Design review of the part built by this model. Coordinates are the model's own, in mm. Face numbers are marked on the shaded views. A direction names the side the tool comes from. Round coordinates to 2 decimals unless told otherwise and drop trailing zeros. Write each loop counter-clockwise with the first axis right and the second up, starting at its lowest first coordinate (ties: lowest second). Pieces come first, ordered by that corner, then holes.
from build123d import *

# Parameters (mm, degrees)
SKETCH1_W               = 6426.2
SKETCH1_H               = 2311.4
BOSS_EXTRUDE1_DEPTH     = 3175
SKETCH2_R               = 763.27
CUT_EXTRUDE1_DEPTH      = 2057.4
CUT_EXTRUDE3_DEPTH      = 7475.536972742
CUT_EXTRUDE3_DEPTH_BACK = 7475.536972742
SKETCH6_W               = 1295.4
SKETCH6_H               = 1651
CUT_EXTRUDE4_DEPTH      = 7523.97968682
CUT_EXTRUDE4_DEPTH_BACK = 7523.97968682
SKETCH7_R               = 444.5
SCALE1_SCALE            = 0.039370079


with BuildPart() as part:
    # Sketch1 → Boss-Extrude1 (new body)
    with BuildSketch(Plane(origin=(0, 0, 0), x_dir=(1, 0, 0), z_dir=(0, 1, 0))):
        with Locations((3156.321169036, 1128.715007899)):
            Rectangle(SKETCH1_W, SKETCH1_H)
    extrude(amount=BOSS_EXTRUDE1_DEPTH)

    # Sketch2 → Cut-Extrude1 (cut)
    with BuildSketch(Plane(origin=(0, 3175, 0), x_dir=(1, 0, 0), z_dir=(0, 1, 0))):
        with Locations(Location((1098.921169036, 1128.715007899, 0), (0, 0, 270))):
            Circle(SKETCH2_R)
        with Locations(Location((3156.321169036, 1128.715007899, 0), (0, 0, 270))):
            Circle(SKETCH2_R)
        with Locations(Location((5213.721169036, 1128.715007899, 0), (0, 0, 270))):
            Circle(SKETCH2_R)
    extrude(amount=-CUT_EXTRUDE1_DEPTH, mode=Mode.SUBTRACT)

    # Sketch6 → Cut-Extrude3 (cut, two sides: drawn at the far end of the back side and taken through both)
    with BuildSketch(Plane.XY.offset(-CUT_EXTRUDE3_DEPTH_BACK)):
        with Locations((3156.321169036, 818.341718397)):
            Rectangle(SKETCH6_W, SKETCH6_H)
        with Locations((5213.721169036, 825.5)):
            Rectangle(SKETCH6_W, SKETCH6_H)
        with Locations((1098.921169036, 825.5)):
            Rectangle(SKETCH6_W, SKETCH6_H)
    extrude(amount=CUT_EXTRUDE3_DEPTH + CUT_EXTRUDE3_DEPTH_BACK, mode=Mode.SUBTRACT)

    # Sketch7 → Cut-Extrude4 (cut, two sides: drawn at the far end of the back side and taken through both)
    with BuildSketch(Plane(origin=(6369.421169036, 0, 0), x_dir=(0, 0, -1), z_dir=(1, 0, 0)).offset(-CUT_EXTRUDE4_DEPTH_BACK)):
        with Locations((1128.715007899, 0)):
            Circle(SKETCH7_R)
    extrude(amount=CUT_EXTRUDE4_DEPTH + CUT_EXTRUDE4_DEPTH_BACK, mode=Mode.SUBTRACT)


with BuildPart() as part_1:
    # Scale1: scaled about (0, 0, 0)
    add(part.part.scale(SCALE1_SCALE))


solid = part_1.part
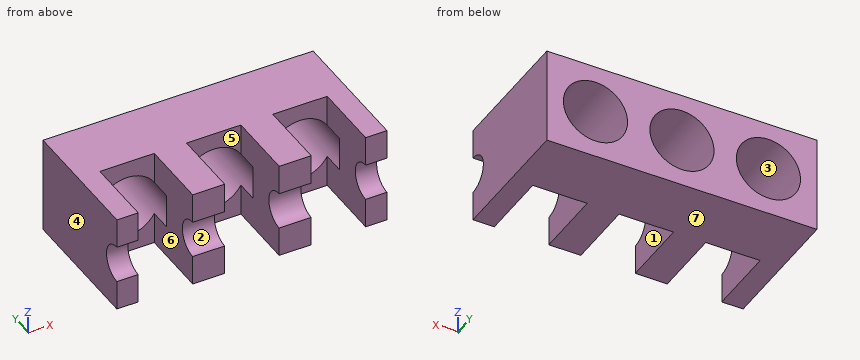
1) Add section B-B on x = 24. State the section outline as (y, z) points.
2) Add section C-C on z = -49. State the section outline as (x, y) points, and give its area (3 significant figures).
3) For the marked faces 1, 2 and 3, list the 3-axis set-ups (+Z, -Z, +X, -X, +Y, -Y) from which the entire face can be reached by the end or side of a thin tool; tool diameter is ignored.
4) For line 1 along X through (y, z) = (60, -22); line 2 along X through (y, z) = (116.5, -63.5); line 3 along Z through (x, y) = (178.5, 9), list the stretches that pass through material, from the lowest coordinate up.
5) Add section A-A on y = 60. State the section outline as (x, z) points.
6) For P1, Ø9, axis at x = 52.5, z = -9, coming from the -Y side; P2, Ø2.5, axis at x = 16, z = -39, coming from the +Y side; P3, Ø5, axis at x = 97.5, z = -51.5, coming from the +Y side; P4, Ø9, axis at x = 119.5, z = -11.5, coming from the -Y side, all flat-tipped, find the tip position at first contact; note any pin that passes through.
7) Add section D-D on x = 91. State the section outline as (y, z) points, and give its area (3 significant figures).
8) The part is to be moulded in two halves that separate along X. For the marked faces 4, 5, 6 and 7, say which applies: pulls with the +X half, pulls with the -X half, needs draft (parallel to the pull), parting line crosses it, or undercut.
Computed:
1. outline: (65, -89.94) - (125, -89.94) - (125, -67.5) - (65, -67.5) - close; (65, -21.38) - (125, -21.38) - (125, 1.06) - (65, 1.06) - close
2. outline: (-2.24, 16.89) - (17.76, 16.89) - (17.76, 44) - (13.56, 44) - (13.56, 125) - (-2.24, 125) - close; (68.76, 16.89) - (98.76, 16.89) - (98.76, 44) - (94.56, 44) - (94.56, 125) - (72.97, 125) - (72.97, 44) - (68.76, 44) - close; (149.76, 16.89) - (179.76, 16.89) - (179.76, 44) - (175.56, 44) - (175.56, 125) - (153.97, 125) - (153.97, 44) - (149.76, 44) - close; (230.76, 16.89) - (250.76, 16.89) - (250.76, 125) - (234.97, 125) - (234.97, 44) - (230.76, 44) - close
2. area: 8,770 mm2
3. face 1: +Z, -Z, -Y
3. face 2: +X, -X, -Y
3. face 3: +Y
4. line 1: x = -2.24 to 17.76, 68.76 to 98.76, 149.76 to 179.76, 230.76 to 250.76
4. line 2: x = -2.24 to 20.03, 66.49 to 101.03, 147.49 to 182.03, 228.49 to 250.76
4. line 3: z = -89.94 to -59.45, -29.43 to 1.06
5. outline: (-2.24, -89.94) - (17.76, -89.94) - (17.76, -60.34) arc R30.05 cw to (17.76, -28.54) - (17.76, 1.06) - (-2.24, 1.06) - close; (68.76, -89.94) - (98.76, -89.94) - (98.76, -60.34) arc R30.05 cw to (98.76, -28.54) - (98.76, 1.06) - (68.76, 1.06) - (68.76, -28.54) arc R30.05 cw to (68.76, -60.34) - close; (149.76, -89.94) - (179.76, -89.94) - (179.76, -60.34) arc R30.05 cw to (179.76, -28.54) - (179.76, 1.06) - (149.76, 1.06) - (149.76, -28.54) arc R30.05 cw to (149.76, -60.34) - close; (230.76, -89.94) - (250.76, -89.94) - (250.76, 1.06) - (230.76, 1.06) - (230.76, -28.54) arc R30.05 cw to (230.76, -60.34) - close
6. P1: stops at y = 65
6. P2: stops at y = 44
6. P3: stops at y = 125
6. P4: stops at y = 64.72
7. outline: (0, -89.94) - (125, -89.94) - (125, 1.06) - (0, 1.06) - (0, -26.94) arc R17.5 cw to (0, -61.94) - close
7. area: 10,900 mm2
8. face 4: pulls with the -X half
8. face 5: undercut
8. face 6: undercut
8. face 7: needs draft
